from build123d import *

# Parameters (mm, degrees)
PAD005_DEPTH    = 4
PAD_DEPTH       = 10
POCKET_DEPTH    = 4.5
POCKET001_DEPTH = 1
SKETCH002_R     = 2.5
PAD004_DEPTH    = 2
SKETCH003_R     = 1.5
POCKET002_DEPTH = 3.501
SKETCH009_W     = 10.607274
SKETCH009_H     = 4.434788
POCKET003_DEPTH = 5
SKETCH010_W     = 7.64298
SKETCH010_H     = 5.328556
POCKET004_DEPTH = 5


with BuildPart() as usb_c_cutter:
    # Sketch008 → Pad005 (new body)
    with BuildSketch(Plane(origin=(0, 0, 0), x_dir=(0, -1, 0), z_dir=(-1, 0, 0))):
        with BuildLine():
            Line((2.535801, 11.911979), (12.347588, 11.911979))
            ThreePointArc((14.347588, 9.911979), (13.761802, 11.326192), (12.347588, 11.911979))
            Line((14.347588, 9.911979), (14.347588, 3.866895))
            ThreePointArc((12.347588, 1.866895), (13.761802, 2.452682), (14.347588, 3.866895))
            Line((12.347588, 1.866895), (2.535801, 1.866895))
            ThreePointArc((0.535801, 3.866895), (1.121588, 2.452682), (2.535801, 1.866895))
            Line((0.535801, 3.866895), (0.535801, 9.911979))
            ThreePointArc((2.535801, 11.911979), (1.121588, 11.326192), (0.535801, 9.911979))
        make_face()
    extrude(amount=-PAD005_DEPTH)


with BuildPart() as usb_c_cutter_1:
    # Body002 placement: moved
    add(usb_c_cutter.part.moved(Location((-26, 0, 0))))


with BuildPart() as body_pocketed:
    # Sketch001 → Pad (new body)
    with BuildSketch(Plane.XY):
        with BuildLine():
            Line((-20.2, 25.5), (20.2, 25.5))
            ThreePointArc((25.5, 20.2), (23.947666, 23.947666), (20.2, 25.5))
            Line((25.5, 20.2), (25.5, -20.2))
            ThreePointArc((20.2, -25.5), (23.947666, -23.947666), (25.5, -20.2))
            Line((20.2, -25.5), (-20.2, -25.5))
            ThreePointArc((-25.5, -20.2), (-23.947666, -23.947666), (-20.2, -25.5))
            Line((-25.5, -20.2), (-25.5, 20.2))
            ThreePointArc((-20.2, 25.5), (-23.947666, 23.947666), (-25.5, 20.2))
        make_face()
    extrude(amount=PAD_DEPTH)

    # Sketch → Pocket (cut, symmetric)
    with BuildSketch(Plane.XY.offset(6)):
        with BuildLine():
            Line((-20.2, 23.5), (20.2, 23.5))
            ThreePointArc((23.5, 20.2), (22.533452, 22.533452), (20.2, 23.5))
            Line((23.5, 20.2), (23.5, -20.2))
            ThreePointArc((20.2, -23.5), (22.533452, -22.533452), (23.5, -20.2))
            Line((20.2, -23.5), (-20.2, -23.5))
            ThreePointArc((-23.5, -20.2), (-22.533452, -22.533452), (-20.2, -23.5))
            Line((-23.5, -20.2), (-23.5, 20.2))
            ThreePointArc((-20.2, 23.5), (-22.533452, 22.533452), (-23.5, 20.2))
        make_face()
    extrude(amount=POCKET_DEPTH, both=True, mode=Mode.SUBTRACT)

    # Sketch004 (on Face5 of Pocket) → Pocket001 (cut, symmetric)
    with BuildSketch(Plane.XY.offset(10)):
        with BuildLine():
            Line((-20.25, 24.25), (20.25, 24.25))
            ThreePointArc((24.25, 20.25), (23.078427, 23.078427), (20.25, 24.25))
            Line((24.25, 20.25), (24.25, -20.25))
            ThreePointArc((20.25, -24.25), (23.078427, -23.078427), (24.25, -20.25))
            Line((20.25, -24.25), (-20.25, -24.25))
            ThreePointArc((-24.25, -20.25), (-23.078427, -23.078427), (-20.25, -24.25))
            Line((-24.25, -20.25), (-24.25, 20.25))
            ThreePointArc((-20.25, 24.25), (-23.078427, 23.078427), (-24.25, 20.25))
        make_face()
    extrude(amount=POCKET001_DEPTH, both=True, mode=Mode.SUBTRACT)

    # Sketch002 (on Face19 of Pocket) → Pad004 (join)
    with BuildSketch(Plane.XY.offset(1.5)):
        with Locations((-20, 20)):
            Circle(SKETCH002_R)
        with Locations((20, 20)):
            Circle(SKETCH002_R)
        with Locations((20, -20)):
            Circle(SKETCH002_R)
        with Locations((-20, -20)):
            Circle(SKETCH002_R)
    extrude(amount=PAD004_DEPTH)

    # Sketch003 → Pocket002 (cut, through all)
    with BuildSketch(Plane.XY.offset(3.5)):
        with Locations((-20, 20)):
            Circle(SKETCH003_R)
        with Locations((20, 20)):
            Circle(SKETCH003_R)
        with Locations((20, -20)):
            Circle(SKETCH003_R)
        with Locations((-20, -20)):
            Circle(SKETCH003_R)
    extrude(amount=-POCKET002_DEPTH, mode=Mode.SUBTRACT)

    # Cut001: cut USB-C Cutter
    add(usb_c_cutter_1.part, mode=Mode.SUBTRACT)

    # Sketch009 (on Face1 of BaseFeature) → Pocket003 (cut)
    with BuildSketch(Plane(origin=(-25.5, 0, 0), x_dir=(0, -1, 0), z_dir=(-1, 0, 0))):
        with Locations((-7.538411, 8.299654)):
            Rectangle(SKETCH009_W, SKETCH009_H)
    extrude(amount=-POCKET003_DEPTH, mode=Mode.SUBTRACT)

    # Sketch010 (on Face17 of Pocket003) → Pocket004 (cut)
    with BuildSketch(Plane.XZ.offset(25.5)):
        with Locations((-12.587816, 7.350035)):
            Rectangle(SKETCH010_W, SKETCH010_H)
    extrude(amount=-POCKET004_DEPTH, mode=Mode.SUBTRACT)


solid = body_pocketed.part
Part model, mm, in its own coordinate system. A direction names the side the tool comes from. Give positions to 0.01 mm unless a question says otherwise; leave off trailing zeros. Loops run counter-clockwise (first coordinate to the right, second up) from the corner with the lowest first, then second, coordinate; pieces in that order, holes last. Notation, with made-up numbers: M 30,-11 L 53,-11 A12 ccw 53,10 Z; hole C 10,-36.75 d4. An arc over 180 degrees is marked long. Put each result on its own line as item: value. Start each with the question number.
1) Saw through at C-C (x = -0.5). List the corners of the cut face in (y, z).
2) Saw through at A-A (z = 7.25). List the corners of the cut face in (x, y), then the cut area to 3 significant figures.
3) 3-axis set-ups, long thin cutter, end or side, ignore diameter. For faces 1 (the flat face through (-16.409, -25, 7)), 2 (the cylindrical face through (-24.51, -13.75, 2.44)), 3 (the cylindrical face through (17.5, -19.9, 2.5)): which of +Z, -Z, +X, -X, +Y, -Y reach the whole face in a straight line?
4) Saw through at B-B (z = 2.5). State how many separate pieces and enclosed holes the cut face has, then the cut area to 3 significant figures.
5) Flat gauge pins, fed straight in: pin 1 (4 mm diameter, centred on x = -3, y = -9.5, fed in from +Z); pin 2 (1.6 mm diameter, centred on x = -12, y = -24.5, fed in from +Z); pin 3 (0.6 mm diameter, centred on y = -24, z = 6, fed in from +X); pin 4 (1.8 mm diameter, centred on x = 20, y = -20, fed in from -Z). Where does each tip first touch, or does it go through?
6) Probe probe 1 along Y at (x, z) = (20, 0.85); probe 2 along X at (y, z) = (20, 7). List the from-to ranges inside material, lowest first.
7) Pull direction Y, two halves, no side cores. Call faces 4 (the cylindrical face through (23.906, -23.989, 4.93)), 5 (the cylindrical face through (-21.11, 21.01, 1.77)), 6 (the flat face through (-25, 1, 10)), 7 (the cylindrical face through (18.89, -18.99, 1.77)): +Y half, -Y half, draft (parallel to the pull), parting line (faces both ways), or undercut.
8) Saw through at D-D (y = -5.5). List the corners of the cut face in (x, z).
Numbers:
1. outline: M -25.5,0 L 25.5,0 L 25.5,10 L 24.25,10 L 24.25,9 L 23.5,9 L 23.5,1.5 L -23.5,1.5 L -23.5,9 L -24.25,9 L -24.25,10 L -25.5,10 Z
2. outline: M -25.5,-20.2 A5.3 ccw -20.2,-25.5 L -16.41,-25.5 L -16.41,-23.5 L -20.2,-23.5 A3.3 cw -23.5,-20.2 L -23.5,-14.35 L -25.5,-14.35 Z; M -25.5,-0.54 L -23.5,-0.54 L -23.5,2.23 L -25.5,2.23 Z; M -25.5,12.84 L -23.5,12.84 L -23.5,20.2 A3.3 cw -20.2,23.5 L 20.2,23.5 A3.3 cw 23.5,20.2 L 23.5,-20.2 A3.3 cw 20.2,-23.5 L -8.77,-23.5 L -8.77,-25.5 L 20.2,-25.5 A5.3 ccw 25.5,-20.2 L 25.5,20.2 A5.3 ccw 20.2,25.5 L -20.2,25.5 A5.3 ccw -25.5,20.2 Z
2. area: 313 mm^2
3. face 1: +Z, -Y
3. face 2: +Z, -X
3. face 3: +Z
4. separate pieces: 5
4. enclosed holes: 4
4. area: 402 mm^2
5. pin 1: z = 1.5
5. pin 2: z = 4.69
5. pin 3: x = 24.18
5. pin 4: through
6. probe 1: -25.5 to -21.5, -18.5 to 18.5, 21.5 to 25.5
6. probe 2: -25.5 to -23.5, 23.5 to 25.5
7. face 4: -Y half
7. face 5: undercut
7. face 6: draft
7. face 7: undercut
8. outline: M -25.5,0 L 25.5,0 L 25.5,10 L 24.25,10 L 24.25,9 L 23.5,9 L 23.5,1.5 L -23.5,1.5 L -23.5,1.87 L -25.5,1.87 Z
